Source: CAD feature listing. Evaluate the final solid. Frame: model axes, mm. Face numbers are marked on the shaded views. A direction names the side the tool comes from. Give positions to 0.01 mm unless a question says otherwise; leave off trailing zeros. Order: outer loops, then holes, each group sorted by start corner. A loop starts at its lowest first (then second) coordinate and runs counter-clockwise, first axis right, second up. Notation, with made-up numbers: M 82,18 L 124,18 A24 ccw 124,29 Z; hole C -35,62 d4. An arc over 180 degrees is marked long. Answer as a JSON object with one key per item and string values. Group by question number.
1. Material intervals for L1, parallel to Z at x = 16.25, y = -5.5; L2, parallel to Z at x = 8, y = -3.25; L3, parallel to X at y = -2.75, z = 14.5, sorted ascending. Write a range as [from, to].
2. Pin query (flat end, axial travel): P1, Ø4, axis at x = 18.5, z = -3.5, coming from the +Y side; P2, Ø2.5, axis at y = -5, z = -6.5, coming from the +X side; P3, Ø1, axis at x = -1, y = -3, coming from the -Z side; P4, Ø1, axis at y = -4, z = -6, coming from the +X side. Return the tip coordinate at first contact, or that it passes through.
3. Section query A-A (x = 3). Output: boundary loops of the cut face in (y, z), plus the area to 3 significant figures.
4. Set-up query: the marked faces 4, 5, 6, 7 and 8. Return all of +Z, -Z, +X, -X, +Y, -Y with unobstructed straight access to the full face (end or side cutting, diameter ignored); none if empty.
5. Pull-direction query (X, two-part tool) for the marked faces 1, 2 and 3; classes: +X half, -X half, draft (parallel to the pull), parting line (faces both ways), or undercut.
6. Section query B-B (z = 9). Output: boundary loops of the cut face in (x, y).
7. Section query C-C (x = 8.25). Output: boundary loops of the cut face in (y, z).
from build123d import *

# Parameters (mm, degrees)
BOSS_EXTRUDE6_DEPTH = 4
BOSS_EXTRUDE7_DEPTH = 4
FILLET5_R           = 0.5
BOSS_EXTRUDE8_DEPTH = 4
BOSS_EXTRUDE9_START = -4
BOSS_EXTRUDE9_DEPTH = 4
FILLET6_R           = 0.5


with BuildPart() as part:
    # Sweep1: sweep along a path in Sketch2path
    with BuildLine(Plane.XY) as sweep1_path:
        Line((17.522352454, -2.291938404), (13.826834324, -0.761204675))
        ThreePointArc((13.826834324, -0.761204675), (11.95090322, -0.192147196), (10, 0))
        Line((10, 0), (0, 0))
    # Sketch3 → Sweep1 (sweep)
    with BuildSketch(Plane(origin=(0, 0, 0), x_dir=(0, 0, -1), z_dir=(1, 0, 0))):
        with BuildLine():
            Line((-16.65, -4), (-16.65, 4))
            ThreePointArc((-16.65, 4), (-15.478427125, 6.828427125), (-12.65, 8))
            Line((-12.65, 8), (12.65, 8))
            ThreePointArc((12.65, 8), (15.478427125, 6.828427125), (16.65, 4))
            Line((16.65, 4), (16.65, -4))
            ThreePointArc((16.65, -4), (15.478427125, -6.828427125), (12.65, -8))
            Line((12.65, -8), (-12.65, -8))
            ThreePointArc((-12.65, -8), (-15.478427125, -6.828427125), (-16.65, -4))
        make_face()
        with BuildLine():
            Line((-15.65, -4), (-15.65, 4))
            ThreePointArc((-15.65, 4), (-14.771320344, 6.121320344), (-12.65, 7))
            Line((-12.65, 7), (12.65, 7))
            ThreePointArc((12.65, 7), (14.771320344, 6.121320344), (15.65, 4))
            Line((15.65, 4), (15.65, -4))
            ThreePointArc((15.65, -4), (14.771320344, -6.121320344), (12.65, -7))
            Line((12.65, -7), (-12.65, -7))
            ThreePointArc((-12.65, -7), (-14.771320344, -6.121320344), (-15.65, -4))
        make_face(mode=Mode.SUBTRACT)
    sweep(path=sweep1_path.line)



with BuildPart() as body_2:
    # Sketch18 → Boss-Extrude6 (new, symmetric)
    with BuildSketch(Plane.ZY):
        with BuildLine():
            Line((-11.65, 5), (0, 5))
            Line((0, 5), (0, 6))
            Line((0, 6), (-11.65, 6))
            ThreePointArc((-11.65, 6), (-13.064213562, 5.414213562), (-13.65, 4))
            Line((-13.65, 4), (-13.65, 0))
            Line((-13.65, 0), (-12.65, 0))
            Line((-12.65, 0), (-12.65, 4))
            ThreePointArc((-12.65, 4), (-12.357106781, 4.707106781), (-11.65, 5))
        make_face()
    extrude(amount=BOSS_EXTRUDE6_DEPTH, both=True)

    # Mirror6: body 2 across plane


with BuildPart() as body_2_1:
    add(body_2.part)
    add(body_2.part.mirror(Plane.XY))

    # Mirror7: body 2 across plane


with BuildPart() as body_2_2:
    add(body_2_1.part)
    add(body_2_1.part.mirror(Plane(origin=(-4, 0, 0), x_dir=(0, 0, 1), z_dir=(0, -1, 0))))


with BuildPart() as part_1:
    add(part.part)

    add(body_2_2.part)  # Boss-Extrude7 merges body 2
    # Sketch19 → Boss-Extrude7 (add)
    with BuildSketch(Plane.ZY):
        with BuildLine():
            Line((-15.65, -4), (-15.65, 4))
            ThreePointArc((-15.65, 4), (-14.771320344, 6.121320344), (-12.65, 7))
            Line((-12.65, 7), (12.65, 7))
            ThreePointArc((12.65, 7), (14.771320344, 6.121320344), (15.65, 4))
            Line((15.65, 4), (15.65, -4))
            ThreePointArc((15.65, -4), (14.771320344, -6.121320344), (12.65, -7))
            Line((12.65, -7), (-12.65, -7))
            ThreePointArc((-12.65, -7), (-14.771320344, -6.121320344), (-15.65, -4))
        make_face()
        with BuildLine():
            Line((-13.65, -4), (-13.65, 4))
            ThreePointArc((-13.65, 4), (-13.064213562, 5.414213562), (-11.65, 6))
            Line((-11.65, 6), (11.65, 6))
            ThreePointArc((11.65, 6), (13.064213562, 5.414213562), (13.65, 4))
            Line((13.65, 4), (13.65, -4))
            ThreePointArc((13.65, -4), (13.064213562, -5.414213562), (11.65, -6))
            Line((11.65, -6), (-11.65, -6))
            ThreePointArc((-11.65, -6), (-13.064213562, -5.414213562), (-13.65, -4))
        make_face(mode=Mode.SUBTRACT)
    extrude(amount=-BOSS_EXTRUDE7_DEPTH)

    # Fillet5
    fillet5_edges = [part_1.edges().sort_by_distance(p)[0] for p in [
        (4, -6.121320344, -14.771320344),
        (4, 0, -15.65),
        (4, 6.121320344, -14.771320344),
        (4, 7, 0),
        (4, 6.121320344, 14.771320344),
        (4, 0, 15.65),
        (4, -6.121320344, 14.771320344),
        (4, -7, 0),
        (-4, 0, -13.65),
        (-4, 6, 0),
        (-4, 5.414213562, 13.064213562),
        (-4, -5.414213562, -13.064213562),
        (4, 5, 0),
        (4, 0, -12.65),
        (-4, -6, 0),
        (-4, -5.414213562, 13.064213562),
        (-4, 0, 13.65),
        (-4, 5.414213562, -13.064213562),
        (4, 4.707106781, -12.357106781),
        (4, -5, 0),
        (4, -4.707106781, 12.357106781),
        (4, 0, 12.65),
        (4, 4.707106781, 12.357106781),
        (4, -4.707106781, -12.357106781),
    ]]
    fillet(fillet5_edges, radius=FILLET5_R)



with BuildPart() as body_2_2_1:
    # Sketch20 → Boss-Extrude8 (new, symmetric)
    with BuildSketch(Plane(origin=(15.766585942, -6.530733729, 0), x_dir=(0, 0, -1), z_dir=(0.9238795325112864, -0.38268343236509084, 0))):
        with BuildLine():
            ThreePointArc((-11.65, 9.588038999), (-12.357106781, 9.29514578), (-12.65, 8.588038999))
            Line((-12.65, 8.588038999), (-12.65, 4.588038999))
            Line((-12.65, 4.588038999), (-13.65, 4.588038999))
            Line((-13.65, 4.588038999), (-13.65, 8.588038999))
            ThreePointArc((-13.65, 8.588038999), (-13.064213562, 10.002252561), (-11.65, 10.588038999))
            Line((-11.65, 10.588038999), (0, 10.588038999))
            Line((0, 10.588038999), (0, 9.588038999))
            Line((0, 9.588038999), (-11.65, 9.588038999))
        make_face()
    extrude(amount=BOSS_EXTRUDE8_DEPTH, both=True)

    # Mirror8: body 2 2 across plane


with BuildPart() as body_2_2_2:
    add(body_2_2_1.part)
    add(body_2_2_1.part.mirror(Plane(origin=(1.755766512, 4.238795325, 0), x_dir=(0, 0, 1), z_dir=(0.3826834323650908, 0.9238795325112864, 0))))

    # Mirror9: body 2 2 across plane


with BuildPart() as body_2_2_3:
    add(body_2_2_2.part)
    add(body_2_2_2.part.mirror(Plane.XY))


with BuildPart() as part_2:
    add(part_1.part)

    add(body_2_2_3.part)  # Boss-Extrude9 merges body 2 2
    # Sketch21 → Boss-Extrude9 (add)
    with BuildSketch(Plane(origin=(15.766585942, -6.530733729, 0), x_dir=(0, 0, -1), z_dir=(0.9238795325112864, -0.38268343236509084, 0)).offset(BOSS_EXTRUDE9_START)):
        with BuildLine():
            Line((-15.65, 8.588038999), (-15.65, 0.588038999))
            ThreePointArc((-15.65, 0.588038999), (-14.771320344, -1.533281345), (-12.65, -2.411961001))
            Line((-12.65, -2.411961001), (12.65, -2.411961001))
            ThreePointArc((12.65, -2.411961001), (14.771320344, -1.533281345), (15.65, 0.588038999))
            Line((15.65, 0.588038999), (15.65, 8.588038999))
            ThreePointArc((15.65, 8.588038999), (14.771320344, 10.709359342), (12.65, 11.588038999))
            Line((12.65, 11.588038999), (-12.65, 11.588038999))
            ThreePointArc((-12.65, 11.588038999), (-14.771320344, 10.709359342), (-15.65, 8.588038999))
        make_face()
        with BuildLine():
            Line((-13.65, 8.588038999), (-13.65, 0.588038999))
            ThreePointArc((-13.65, 0.588038999), (-13.064213562, -0.826174564), (-11.65, -1.411961001))
            Line((-11.65, -1.411961001), (11.65, -1.411961001))
            ThreePointArc((11.65, -1.411961001), (13.064213562, -0.826174564), (13.65, 0.588038999))
            Line((13.65, 0.588038999), (13.65, 8.588038999))
            ThreePointArc((13.65, 8.588038999), (13.064213562, 10.002252561), (11.65, 10.588038999))
            Line((11.65, 10.588038999), (-11.65, 10.588038999))
            ThreePointArc((-11.65, 10.588038999), (-13.064213562, 10.002252561), (-13.65, 8.588038999))
        make_face(mode=Mode.SUBTRACT)
    extrude(amount=BOSS_EXTRUDE9_DEPTH)

    # Fillet6
    fillet6_edges = [part_2.edges().sort_by_distance(p)[0] for p in [
        (23.019202363, 0.526127479, 12.357106781),
        (23.131287746, 0.796725529, 0),
        (21.217870584, -3.822672134, 12.65),
        (23.019202363, 0.526127479, -12.357106781),
        (21.217870584, -3.822672134, -12.65),
        (19.304453422, -8.442069796, 0),
        (19.416538804, -8.171471746, 12.357106781),
        (15.628166103, 3.587594938, 12.357106781),
        (13.826834324, -0.761204675, 12.65),
        (12.025502544, -5.110004287, -12.357106781),
        (15.740251485, 3.858192988, 0),
        (12.025502544, -5.110004287, 12.357106781),
        (11.913417162, -5.380602337, 0),
        (15.628166103, 3.587594938, -12.357106781),
        (13.826834324, -0.761204675, -12.65),
        (19.416538804, -8.171471746, -12.357106781),
        (16.169362203, 4.894157902, 14.771320344),
        (13.826834324, -0.761204675, 15.65),
        (11.484306444, -6.416567252, 14.771320344),
        (11.148050297, -7.228361402, 0),
        (11.484306444, -6.416567252, -14.771320344),
        (13.826834324, -0.761204675, -15.65),
        (16.169362203, 4.894157902, -14.771320344),
        (16.50561835, 5.705952053, 0),
    ]]
    fillet(fillet6_edges, radius=FILLET6_R)

    # SurfaceCut1
    split(bisect_by=Plane(origin=(0, -2, 0), x_dir=(1, 0, 0), z_dir=(0, 1, 0)), keep=Keep.BOTTOM)


solid = part_2.part
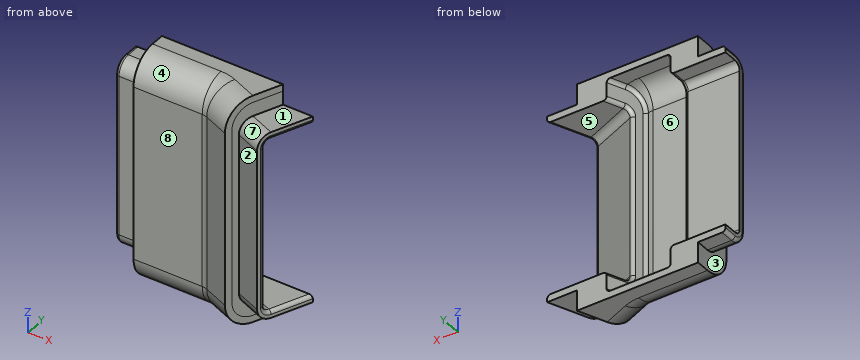
Answer sheet:
{
 "1": {"L1": "[-13.65, -12.65], [12.65, 13.65]", "L2": "[-16.65, -15.65], [15.65, 16.65]", "L3": "[0, 4], [13, 17.33]"},
 "2": {"P1": "y = -7.28", "P2": "x = 14.01", "P3": "z = -13.65", "P4": "through"},
 "3": {"outline": "M -8,-12.65 A4 ccw -4,-16.65 L -2,-16.65 L -2,-12.65 L -4,-12.65 A1 cw -5,-11.65 L -5,11.65 A1 cw -4,12.65 L -2,12.65 L -2,16.65 L -4,16.65 A4 ccw -8,12.65 Z", "area": "117 mm^2"},
 "4": {"face 4": "+Z, -X, -Y", "face 5": "+X, +Y", "face 6": "+Y", "face 7": "+Z, -Y", "face 8": "+Z, -Z, -X, -Y"},
 "5": {"face 1": "draft", "face 2": "undercut", "face 3": "-X half"},
 "6": {"outline": "M -4,-5.5 A0.5 ccw -3.5,-6 L 0,-6 L 0,-8 L 10,-8 A2 cw 10.77,-8.15 L 14.46,-9.68 L 15.23,-7.84 L 18.92,-9.37 L 19.11,-8.9 A0.5 ccw 18.84,-8.25 L 12.38,-5.57 A0.5 ccw 11.72,-5.84 L 11.33,-6.8 A0.5 cw 10.74,-7.09 A3 ccw 10,-7 L 4.5,-7 A0.5 cw 4,-6.5 L 4,-5.5 A0.5 ccw 3.5,-5 L -4,-5 Z"},
 "7": {"outline": "M -8,-12.65 A4 ccw -4,-16.65 L -2,-16.65 L -2,-15.65 L -4,-15.65 A3 cw -7,-12.65 L -7,12.65 A3 cw -4,15.65 L -2,15.65 L -2,16.65 L -4,16.65 A4 ccw -8,12.65 Z"}
}
